Can you work these out from the model? Positions are in its coordinate system, mm. A direction names the side the tool comes from. Give positions to 0.01 mm unless a question says otherwise; leave off trailing zeros. Answer as CSV lines item,"result". Start each with the question number.
1. If we section it at A-A on y = 0: Count the separate pieces of the cut face and the enclosed holes in it, plus the area to 3 significant figures.
2. I'm going to push flat-ended pins straight in: P1, Ø1, axis at y = 10, z = -17, coming from the -X side; P2, Ø1.5, axis at x = 117.5, y = 31.5, coming from the -Z side; P3, Ø5, axis at y = 74.5, z = 7.5, coming from the -X side. Where does each tip first touch, or does it pass through?
3. If we mould it in two halves opening along Z, with no side actions, what happens to faces 1 (the face through (124.923, -39.34, -22.448)), 2 (the face through (-19.527, 148.724, 33.427)), 3 (the face through (123.997, -39.048, -16.589)), 4 (the face through (106.77, -33.62, 31.56))? For each: pulls with the +Z half, pulls with the -Z half, needs draft (parallel to the pull), parting line crosses it, or undercut.
4. On a 3-axis mill with a long thin cutter (end or side, diameter ignored), from which of +Z, -Z, +X, -X, +Y, -Y can I reach the whole of each face in a straight line? I mean faces 5 (the face through (-28.453, 128.13, -10.823)), 6 (the face through (-23, -30, -40)), 7 (the face through (47, -23, 13.333)), 8 (the face through (-23, -30, 40)), 9 (the face through (101.612, -42.131, -22.357)). Say none if no direction works.
5. I need wall thicknesses on line 1 (X direction, y = 28, z = -21); line 2 (Y direction, x = 31.5, z = -16); line 3 (Z direction, x = 129.5, y = 30.5). Which ranges of each line are inside material? Lowest first, please. Write a range as [from, to].
```python
from build123d import *

# Parameters (mm, degrees)
SKETCH1_R             = 150
SKETCH1_R_2           = 110
BOSS_EXTRUDE1_DEPTH   = 40
SKETCH1_R_3           = 50.833333333
SKETCH1_R_4           = 37.5
BOSS_EXTRUDE1_2_DEPTH = 40
SKETCH1_3_R           = 17.5
BOSS_EXTRUDE2_DEPTH   = 13.333333333


with BuildPart() as part:
    # Sketch1 → Boss-Extrude1 (new, symmetric)
    with BuildSketch(Plane.XY):
        Circle(SKETCH1_R)
        Circle(SKETCH1_R_2, mode=Mode.SUBTRACT)
    extrude(amount=BOSS_EXTRUDE1_DEPTH, both=True)



with BuildPart() as body_2:
    # Sketch1 → Boss-Extrude1 2 (new, symmetric)
    with BuildSketch(Plane.XY):
        Circle(SKETCH1_R_3)
        Circle(SKETCH1_R_4, mode=Mode.SUBTRACT)
    extrude(amount=BOSS_EXTRUDE1_2_DEPTH, both=True)


with BuildPart() as part_1:
    add(part.part)

    add(body_2.part)  # Boss-Extrude2 merges body 2
    # Sketch1_3 → Boss-Extrude2 (add, symmetric)
    with BuildSketch(Plane.XY):
        with BuildLine():
            ThreePointArc((110, 0), (77.781745931, 77.781745931), (0, 110))
            ThreePointArc((0, 110), (-77.781745931, -77.781745931), (110, 0))
        make_face()
        with Locations((-56.86317032, -56.86317032)):
            Circle(SKETCH1_3_R, mode=Mode.SUBTRACT)
        with Locations((0, -80.416666667)):
            Circle(SKETCH1_3_R, mode=Mode.SUBTRACT)
        with Locations((56.86317032, -56.86317032)):
            Circle(SKETCH1_3_R, mode=Mode.SUBTRACT)
        with Locations((-80.416666667, 0)):
            Circle(SKETCH1_3_R, mode=Mode.SUBTRACT)
        with Locations((-56.86317032, 56.86317032)):
            Circle(SKETCH1_3_R, mode=Mode.SUBTRACT)
        with BuildLine():
            ThreePointArc((50.833333333, 0), (-35.94459471, -35.94459471), (0, 50.833333333))
            ThreePointArc((0, 50.833333333), (35.94459471, 35.94459471), (50.833333333, 0))
        make_face(mode=Mode.SUBTRACT)
        with Locations((56.86317032, 56.86317032)):
            Circle(SKETCH1_3_R, mode=Mode.SUBTRACT)
        with Locations((80.416666667, 0)):
            Circle(SKETCH1_3_R, mode=Mode.SUBTRACT)
        with BuildLine():
            ThreePointArc((17.5, 80.416666667), (12.374368671, 68.042297996), (0, 62.916666667))
            ThreePointArc((0, 62.916666667), (-17.5, 80.416666667), (0, 97.916666667))
            ThreePointArc((0, 97.916666667), (12.374368671, 92.791035337), (17.5, 80.416666667))
        make_face(mode=Mode.SUBTRACT)
    extrude(amount=BOSS_EXTRUDE2_DEPTH, both=True)

    # Sketch2 → Cut-Revolve2 (revolve, cut)
    with BuildSketch(Plane(origin=(0, 0, 0), x_dir=(0, 0, -1), z_dir=(1, 0, 0)), mode=Mode.PRIVATE) as cut_revolve2_sk:
        Polygon((-40, 150), (-31.132213494, 110), (-40, 110), align=None)
    revolve(cut_revolve2_sk.sketch.rotate(Axis((0, 0, 46.027380227), (0, 0, -1)), 90), axis=Axis((0, 0, 46.027380227), (0, 0, -1)), mode=Mode.SUBTRACT)

    # Sketch2_5 → Cut-Revolve3 (revolve, cut)
    with BuildSketch(Plane(origin=(0, 0, 0), x_dir=(0, 0, -1), z_dir=(1, 0, 0)), mode=Mode.PRIVATE) as cut_revolve3_sk:
        Polygon((31.132213494, 110), (40, 110), (40, 150), align=None)
    revolve(cut_revolve3_sk.sketch.rotate(Axis((0, 0, 46.027380227), (0, 0, -1)), 90), axis=Axis((0, 0, 46.027380227), (0, 0, -1)), mode=Mode.SUBTRACT)

    # Sketch2_7 → Cut-Revolve5 (revolve, cut)
    with BuildSketch(Plane(origin=(0, 0, 0), x_dir=(0, 0, -1), z_dir=(1, 0, 0)), mode=Mode.PRIVATE) as cut_revolve5_sk:
        Polygon((-6.666666667, 150), (-26.666666667, 150), (-22.232773414, 130), (-11.10055992, 130), align=None)
    cut_revolve5 = revolve(cut_revolve5_sk.sketch.rotate(Axis((0, 0, 46.027380227), (0, 0, -1)), 90), axis=Axis((0, 0, 46.027380227), (0, 0, -1)), mode=Mode.SUBTRACT)

    # Mirror1: Cut-Revolve5 across plane
    add(cut_revolve5.mirror(Plane.XY), mode=Mode.SUBTRACT)


solid = part_1.part
```
Computed values:
1,separate pieces,"4"
1,enclosed holes,"0"
1,area,"7,870 mm2"
2,P1,"stops at x = -129.65"
2,P2,"stops at z = -33.88"
2,P3,"stops at x = -131.51"
3,face 1,"undercut"
3,face 2,"needs draft"
3,face 3,"undercut"
3,face 4,"pulls with the +Z half"
4,face 5,"none"
4,face 6,"-Z, +X, -X, +Y, -Y"
4,face 7,"+Z"
4,face 8,"+Z, +X, -X, +Y, -Y"
4,face 9,"-Z"
5,line 1,"x = [-126.95, -106.38], [-42.43, -24.94], [24.94, 42.43], [106.38, 126.95]"
5,line 2,"y = [-126.13, -105.39], [-39.9, -20.35], [20.35, 39.9], [105.39, 126.13]"
5,line 3,"z = [-36.24, -22.91], [-10.43, 10.43], [22.91, 36.24]"
